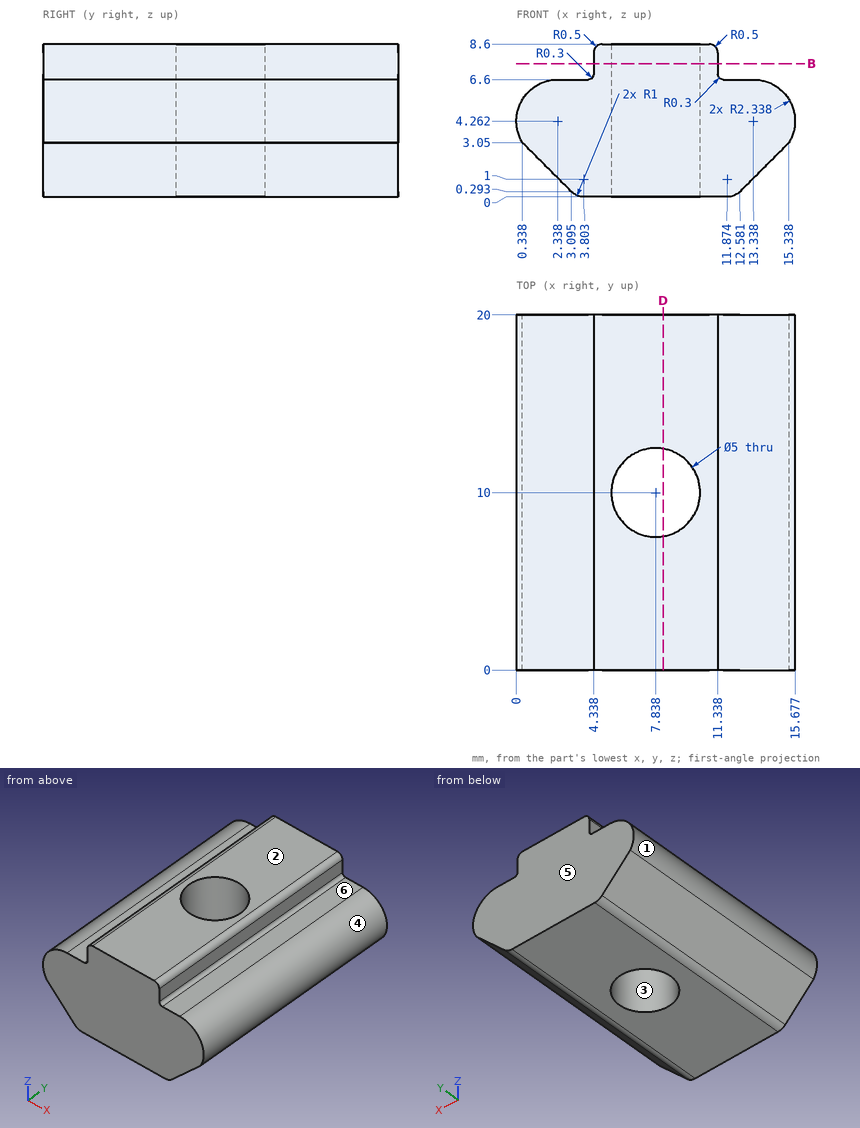
Drawing for the job (mm, zero at the part's lowest x, y, z). A direction names the side the tool comes from. Coordinates: 2 decimals unless noted, no trailing zeros. Order: outer loops, then holes, each group sorted by start corner. A loop starts at its lowest first (then second) coordinate and runs counter-clockwise, first axis right, second up. Notation, with made-up numbers: (59, 9.5) -> (88, 9.5) arc R21 ccw to (88, 44.5) -> close; hole circle Ø3 at (-38, -1). An arc over 180 degrees is marked (long way). One line per item, written item: value.
(1) Slice it at B-B, the plane z = 7.5. List the corners of the cut face in (x, y).
Checked values:
outline: (4.34, 0) -> (11.34, 0) -> (11.34, 20) -> (4.34, 20) -> close; hole circle Ø5 at (7.84, 10)
(2) Tool access for the marked faces 5 and 6: list every direction of +Z, -Z, +X, -X, +Y, -Y with a clear straight run to the whole face (end or side of a thin tool).
Checked values:
face 5: +Z, -Z, +X, -X, +Y
face 6: +Z, +X, +Y, -Y
(3) Probe line 1 (Y direction, x = 8, z = 4.75) (1 decimal); line 2 (X direction, y = 10, z = 7); line 3 (X direction, y = 10, z = 2.5). List the from-to ranges inside material, lowest first. Write a range as [from, to].
Checked values:
line 1: [0, 7.5], [12.5, 20]
line 2: [4.34, 5.34], [10.34, 11.34]
line 3: [0.89, 5.34], [10.34, 14.79]
(4) Drop flat-ended pins along their axis: pin 1 Ø1.5 at (y, z) = (10.5, 1) entering from -X; pin 2 Ø1.9 at (x, y) = (3, 5) entering from +Z; pin 3 Ø0.6 at (y, z) = (12.5, 8) entering from +X; pin 4 Ø3 at (x, y) = (7.84, 10) entering from +Z. Give the stop position or say it passes through.
Checked values:
pin 1: x = 1.64
pin 2: z = 6.6
pin 3: x = 11.34
pin 4: through
(5) Slice it at D-D, the plane x = 8.25. List the corners of the cut face in (y, z) (1 decimal), plus the area to 3 significant figures.
Checked values:
outline: (0, 0) -> (7.5, 0) -> (7.5, 8.6) -> (0, 8.6) -> close; (12.5, 0) -> (20, 0) -> (20, 8.6) -> (12.5, 8.6) -> close
area: 130 mm2
(6) Mould opens along X. For the marked faces 1, 2, 3 and 4 say: pulls with the +X half, pulls with the -X half, needs draft (parallel to the pull), parting line crosses it, or undercut.
Checked values:
face 1: pulls with the -X half
face 2: needs draft
face 3: undercut
face 4: pulls with the +X half
